Read the model definition and answer for the solid it produces. Units are mm, in the model's axes. Face numbers are marked on the shaded views. A direction names the side the tool comes from. Coordinates: 2 decimals unless noted, no trailing zeros. Write each loop counter-clockwise with the first axis right and the second up, starting at its lowest first coordinate (ties: lowest second). Pieces come first, ordered by that corner, then holes.
(1) Which of the six approach directions +Z, -Z, +X, -X, +Y, -Y give full straight-line access (tool end or side, diameter ignored) to the marked faces 1 and 2?
(2) Section D-D on z = 21 is taken. Write down the section's boundary in (x, y), then the cut area to 3 significant figures.
(3) The mould has two halves that part along Z. Classify the marked faces 3, 4, 5 and 6: +Z half, -Z half, draft (parallel to the pull), parting line (faces both ways), or undercut.
(4) Section B-B on z = 0 is taken. Write down the section's boundary in (x, y), then the cut area to 4 significant figures.
(5) Given pin 1 (4 mm diameter, centred on x = -55, z = -21, fed in from -Y); pin 2 (2.5 mm diameter, centred on y = 4, z = -27, fed in from +X); pin 3 (4 mm diameter, centred on y = 5.5, z = 12.5, fed in from +X), each flat-ended and moving along its own axis, determine where each tip first touches the part or whether it passes through.
(6) Find the intervals of material crossed by probe 1 along Z at (x, y) = (94.5, 12); probe 2 along X at (y, z) = (4.75, -9.5); probe 3 along X at (y, z) = (4.25, -10.5), in increasing order.
(7) Section C-C on x = 85 is taken. Write down the section's boundary in (y, z).
(8) Section A-A on y = 10 is taken. Write down the section's boundary in (x, z).
from build123d import *

# Parameters (mm, degrees)
BOSS_EXTRUDE1_DEPTH          = 15
TAP_DRILL_FOR_M30X2_0_TAP1_D = 28


with BuildPart() as part:
    # Sketch1 → Boss-Extrude1 (new body)
    with BuildSketch(Plane(origin=(0, 0, 0), x_dir=(1, 0, 0), z_dir=(0, 1, 0))):
        with BuildLine():
            Line((-114.776877535, 40), (95.223122465, 40))
            ThreePointArc((95.223122465, 40), (135.223122465, 0), (95.223122465, -40))
            Line((95.223122465, -40), (-114.776877535, -40))
            Line((-114.776877535, -40), (-114.776877535, 40))
        make_face()
        with BuildLine():
            Line((95.223122465, 30), (95.223122465, 25))
            ThreePointArc((95.223122465, 25), (70.223122465, 0), (95.223122465, -25))
            Line((95.223122465, -25), (95.223122465, -30))
            ThreePointArc((95.223122465, -30), (125.223122465, 0), (95.223122465, 30))
        make_face(mode=Mode.SUBTRACT)
    extrude(amount=BOSS_EXTRUDE1_DEPTH)

    # Tap Drill for M30x2.0 Tap1 (through all)
    with Locations(Plane(origin=(0, 15, 0), x_dir=(1, 0, 0), z_dir=(0, 1, 0))):
        with Locations((10.223122465, 0)):
            Hole(TAP_DRILL_FOR_M30X2_0_TAP1_D / 2)


solid = part.part
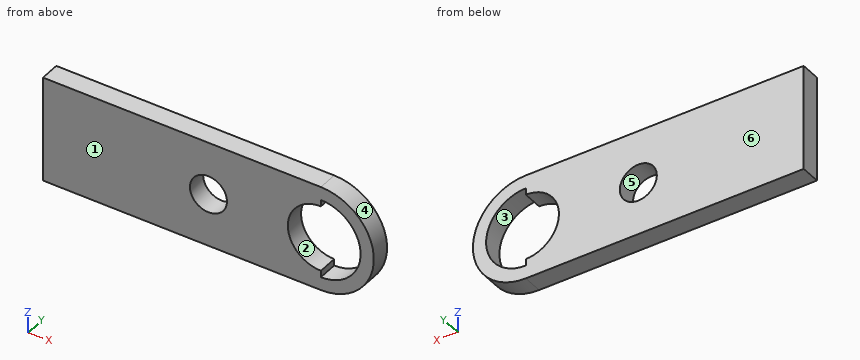
Response:
1. face 1: +Z, -Z, +X, -X, -Y
1. face 2: +Y, -Y
2. outline: (-114.78, 0) - (81.66, 0) - (81.66, 15) - (-114.78, 15) - close; (116.65, 0) - (129.27, 0) - (129.27, 15) - (116.65, 15) - close
2. area: 3,140 mm2
3. face 3: undercut
3. face 4: parting line
3. face 5: undercut
3. face 6: draft
4. outline: (-114.78, 0) - (-3.78, 0) - (-3.78, 15) - (-114.78, 15) - close; (24.22, 0) - (70.22, 0) - (70.22, 15) - (24.22, 15) - close; (125.22, 0) - (135.22, 0) - (135.22, 15) - (125.22, 15) - close
4. area: 2,505 mm2
5. pin 1: stops at y = 0
5. pin 2: stops at x = 125.83
5. pin 3: stops at x = 133.82
6. probe 1: z = -40 to -24.99, 24.99 to 40
6. probe 2: x = -114.78 to -0.06, 20.51 to 72.1, 123.68 to 134.08
6. probe 3: x = -114.78 to 0.96, 19.48 to 72.54, 123.33 to 133.82
7. outline: (0, -40) - (15, -40) - (15, -22.81) - (0, -22.81) - close; (0, 22.81) - (15, 22.81) - (15, 40) - (0, 40) - close
8. outline: (-114.78, -40) - (95.22, -40) arc R40 ccw to (95.22, 40) - (-114.78, 40) - close; hole circle Ø28 at (10.22, 0); hole (95.22, -30) arc R30 ccw to (95.22, 30) - (95.22, 25) arc R25 ccw to (95.22, -25) - close
